Read the model definition and answer for the solid it produces. Units are mm, in the model's axes. Give positions to 0.01 mm unless a question says otherwise; leave off trailing zeros. Write each loop counter-clockwise with the first axis right and the second up, starting at its lowest first coordinate (ties: lowest second). Pieces come first, ordered by that corner, then holes. Notation, with made-up numbers: (42.5, 9.5) -> (96.5, 9.5) arc R23 ccw to (96.5, 32.5) -> close; hole circle Ø1 at (29.5, -30.5). An arc over 180 degrees is marked (long way). Write item = value, one per line.
Autodesk Inventor part; units mm, degrees
ref_plane "YZ Plane" through (0, 0, 0) normal (1, 0, 0) x (0, 1, 0)
ref_plane "XZ Plane" through (0, 0, 0) normal (0, 1, 0) x (-1, 0, 0)
ref_plane "XY Plane" through (0, 0, 0) normal (0, 0, 1) x (1, 0, 0)
sketch "Sketch1" plane through (0, 0, 0) normal (0, 0, 1) x (1, 0, 0)
  line L0 (-40, 40) -> (40, 40)
  line L1 (40, 40) -> (40, -40)
  line L2 (40, -40) -> (-40, -40)
  line L3 (-40, -40) -> (-40, 40)
  point P0 (0, 0)
  point P1 (0, 40)
  point P2 (-40, 0)
  dimension "d0" = 80
extrude "Extrusion1" add sketch "Sketch1" along normal blind 15
sketch "Sketch2" plane through (0, 0, 15) normal (0, 0, 1) x (1, 0, 0)
  line L0 (-35.75, 35.75) -> (35.75, 35.75)
  line L1 (35.75, 35.75) -> (35.75, -35.75)
  line L2 (35.75, -35.75) -> (-35.75, -35.75)
  line L3 (-35.75, -35.75) -> (-35.75, 35.75)
  point P0 (0, 0)
  point P1 (0, 35.75)
  point P2 (-35.75, 0)
  dimension "d3" = 71.5
hole "Hole1" at (-35.75, 35.75, 15) at (35.75, 35.75, 15) at (-35.75, -35.75, 15) at (35.75, -35.75, 15) direction (0, 0, -1) diameter 4.4 end through all
fillet "Fillet1" radius 2 4 edges at (-40, 40, 7.5) (40, 40, 7.5) (40, -40, 7.5) (-40, -40, 7.5)
properties part number "FAN SPACE MODEL"
(1) For a pull along Y with two mould halves and no side action, classify faces 1 (the cylindrical face through (-39.43, -39.4, 7.6)), 2 (the cylindrical face through (39.43, 39.4, 7.6)), 3 (the flat face through (-1, 1, 15)), 4 (the cylindrical face through (37.898, -35.273, 7.395)) as released by +Y, released by -Y, zero draft, split by the parting line, or undercut.
Checks:
face_1 = released by -Y
face_2 = released by +Y
face_3 = zero draft
face_4 = undercut
(2) The part is cut by section A-A on y = -35.75. Determine the outline of the cut face in (x, z).
Checks:
outline = (-40, 0) -> (-37.95, 0) -> (-37.95, 15) -> (-40, 15) -> close; (-33.55, 0) -> (33.55, 0) -> (33.55, 15) -> (-33.55, 15) -> close; (37.95, 0) -> (40, 0) -> (40, 15) -> (37.95, 15) -> close
(3) Consider L1, parallel to Y at x = -35.75, z = 10.25. Determine where the line is inside the solid, lowest interval first.
Checks:
L1 = -40 to -37.95, -33.55 to 33.55, 37.95 to 40
